Check sheet for the drawn part. Datum: minimum x, y, z corner. Units: mm. Give positions to 0.01 mm unless a question says otherwise; leave off trailing zeros. Loops run counter-clockwise (first coordinate to the right, second up) from the corner with the lowest first, then second, coordinate; pieces in that order, holes last. Notation, with made-up numbers: (-21.75, 46) - (4.25, 46) arc R12 ccw to (4.25, 68) - close; hole circle Ø6 at (61, 86). An arc over 180 degrees is marked (long way). Answer in a Markdown table with one row per item.
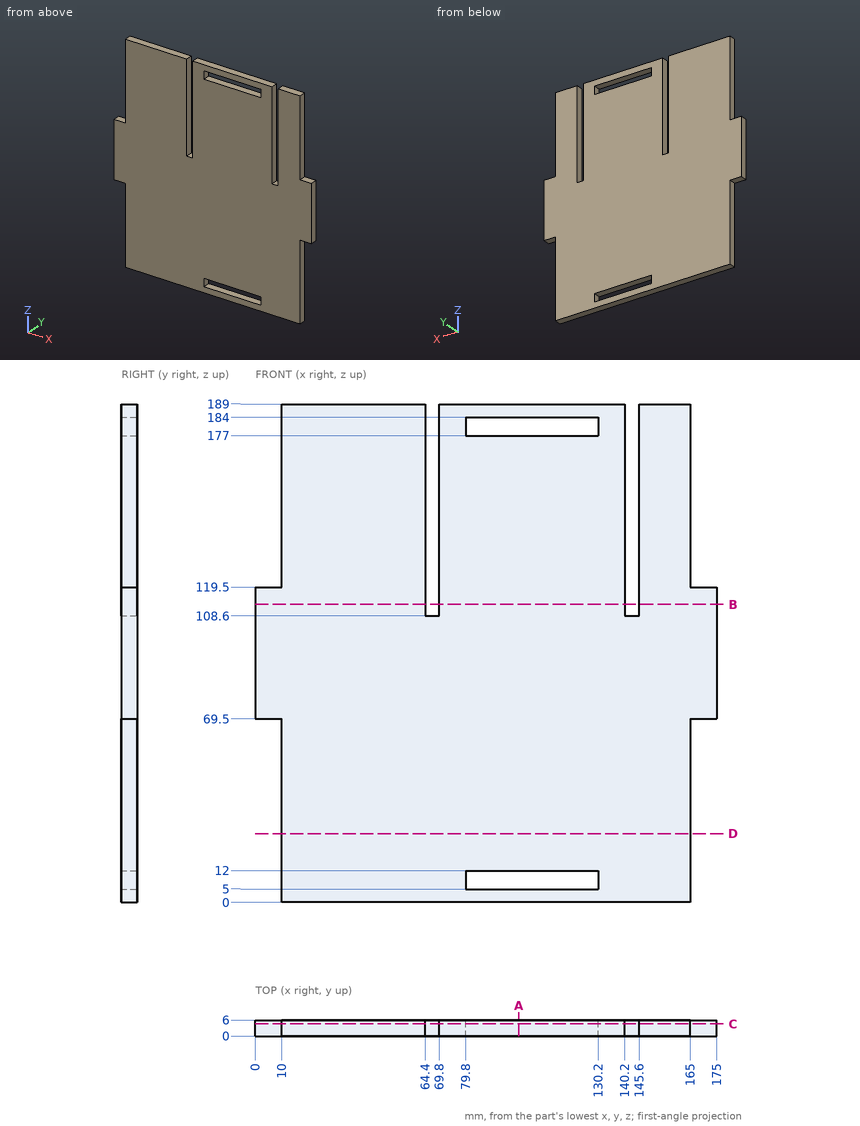
Q1. Thickness scan on line 1 (Z direction, x = 93, y = 3.6); line 2 (X direction, y = 1.5, z = 122); line 3 (X direction, y = 2.1, z = 119). Record the ranges inside material, lowest first.
Completed:
| item | result |
|---|---|
| line 1 | 0 to 5, 12 to 177, 184 to 189 |
| line 2 | 10 to 64.4, 69.8 to 140.2, 145.6 to 165 |
| line 3 | 0 to 64.4, 69.8 to 140.2, 145.6 to 175 |
Q2. Sectioned sample at C-C (y = 4.6). Record the cut outline in (x, z), and give its area (3 significant figures).
Completed:
| item | result |
|---|---|
| outline | (0, 69.5) - (10, 69.5) - (10, 0) - (165, 0) - (165, 69.5) - (175, 69.5) - (175, 119.5) - (165, 119.5) - (165, 189) - (145.6, 189) - (145.6, 108.6) - (140.2, 108.6) - (140.2, 189) - (69.8, 189) - (69.8, 108.6) - (64.4, 108.6) - (64.4, 189) - (10, 189) - (10, 119.5) - (0, 119.5) - close; hole (79.8, 5) - (130.2, 5) - (130.2, 12) - (79.8, 12) - close; hole (79.8, 177) - (130.2, 177) - (130.2, 184) - (79.8, 184) - close |
| area | 28,700 mm^2 |
Q3. Go/stop test with flat-tipped pins: P1, Ø2, axis at y = 2.5, z = 148.5, coming from the +X side; P2, Ø3, axis at y = 2.5, z = 138, coming from the -X side; P3, Ø1.8, axis at x = 7, y = 3.5, coming from the -Z side. Record where each tip stops, or that it passes through.
Completed:
| item | result |
|---|---|
| P1 | x = 165 |
| P2 | x = 10 |
| P3 | z = 69.5 |
Q4. Sectioned sample at B-B (z = 113). Record the cut outline in (x, y), and give its area (3 significant figures).
Completed:
| item | result |
|---|---|
| outline | (0, 0) - (64.4, 0) - (64.4, 6) - (0, 6) - close; (69.8, 0) - (140.2, 0) - (140.2, 6) - (69.8, 6) - close; (145.6, 0) - (175, 0) - (175, 6) - (145.6, 6) - close |
| area | 985 mm^2 |
Q5. Sectioned sample at A-A (x = 100). Record the cut outline in (y, z).
Completed:
| item | result |
|---|---|
| outline | (0, 0) - (6, 0) - (6, 5) - (0, 5) - close; (0, 12) - (6, 12) - (6, 177) - (0, 177) - close; (0, 184) - (6, 184) - (6, 189) - (0, 189) - close |
Q6. Sectioned sample at D-D (z = 26). Record the cut outline in (x, y), and give its area (3 significant figures).
Completed:
| item | result |
|---|---|
| outline | (10, 0) - (165, 0) - (165, 6) - (10, 6) - close |
| area | 930 mm^2 |
